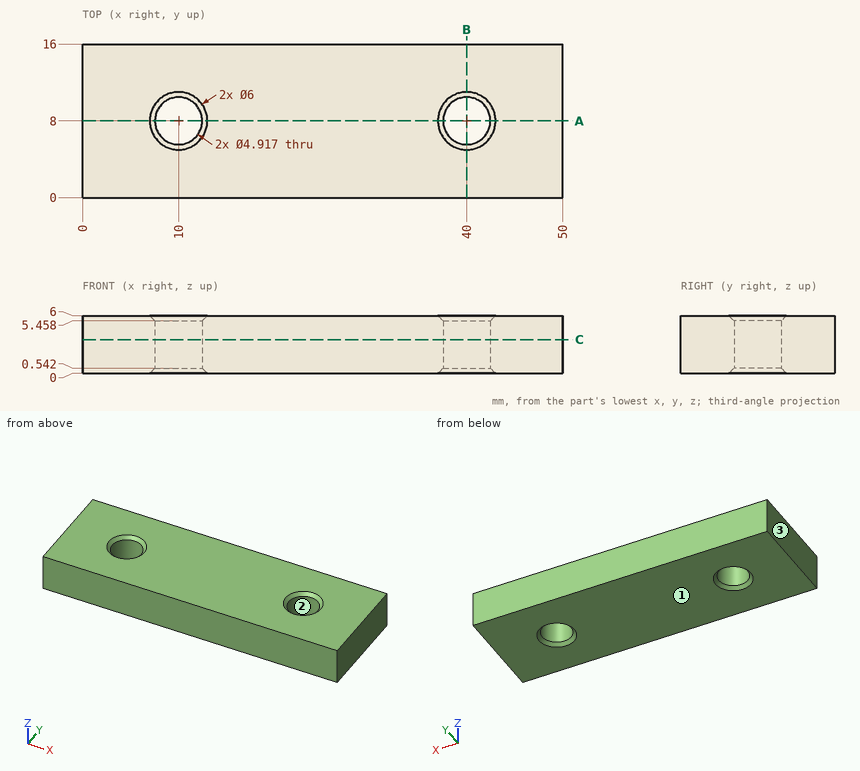
The drawing under review shows one solid part. Ordinate dimensions are in mm from its lowest x, y, z. Round coordinates to 2 decimals unless told otherwise and drop trailing zeros. Loops run counter-clockwise (first coordinate to the right, second up) from the corner with the lowest first, then second, coordinate; pieces in that order, holes last. Notation, with made-up numbers: (80.25, 0) - (122.25, 0) arc R6 ccw to (122.25, 11) - close; hole circle Ø5 at (74, 65.25). An arc over 180 degrees is marked (long way). One line per item, written item: value. Start each with the question number.
1) To check wall thickness, follow L1, parallel to X at y = 8, z = 3.4; L2, parallel to Y at x = 10, z = 3.4; L3, parallel to X at y = 6.75, z = 4.3 (1 decimal). State the ranges of each line that lie inside material, in increasing order. Write a range as from..to.
2) Insertion check: pin 1 Ø4 at (x, y) = (10, 8) entering from +Z. The pin has a flat end and moves straight along its axis. Give the tip position at first contact, or say it passes through.
3) Consider section B-B on x = 40. Give the boundary of the cut face in (y, z).
4) Draft analysis for pull direction X (two halves, no side actions). For the marked faces 1, 2 and 3, state which applies: +X half, -X half, draft (parallel to the pull), parting line (faces both ways), or undercut.
5) Consider section A-A on y = 8. Give the boundary of the cut face in (x, z).
6) Consider section C-C on z = 3.5. Give the boundary of the cut face in (x, y), then the cut area to 3 significant figures.
Reported:
1. L1: x = 0..7.54, 12.46..37.54, 42.46..50
1. L2: y = 0..5.54, 10.46..16
1. L3: x = 0..7.9, 12.1..37.9, 42.1..50
2. pin 1: passes through
3. outline: (0, 0) - (5, 0) - (5.54, 0.54) - (5.54, 5.46) - (5, 6) - (0, 6) - close; (10.46, 0.54) - (11, 0) - (16, 0) - (16, 6) - (11, 6) - (10.46, 5.46) - close
4. face 1: draft
4. face 2: undercut
4. face 3: -X half
5. outline: (0, 0) - (7, 0) - (7.54, 0.54) - (7.54, 5.46) - (7, 6) - (0, 6) - close; (12.46, 0.54) - (13, 0) - (37, 0) - (37.54, 0.54) - (37.54, 5.46) - (37, 6) - (13, 6) - (12.46, 5.46) - close; (42.46, 0.54) - (43, 0) - (50, 0) - (50, 6) - (43, 6) - (42.46, 5.46) - close
6. outline: (0, 0) - (50, 0) - (50, 16) - (0, 16) - close; hole circle Ø4.92 at (10, 8); hole circle Ø4.92 at (40, 8)
6. area: 762 mm^2
